Could you check a few things on this model? Use its own coordinates, in mm. Face numbers are marked on the shaded views. A direction names the side the tool comes from. Give positions to 0.01 mm unless a question says otherwise; leave off trailing zeros. Loops run counter-clockwise (first coordinate to the right, second up) from the corner with the lowest first, then second, coordinate; pieces in that order, holes last. Notation, with made-up numbers: (-7.5, -22.5) - (33.5, -22.5) arc R10 cw to (33.5, -13.5) - close; hole circle Ø11 at (38.5, 61.5). An arc over 180 degrees is marked (long way). Answer in a Markdown table with one row per item. Add a question column.
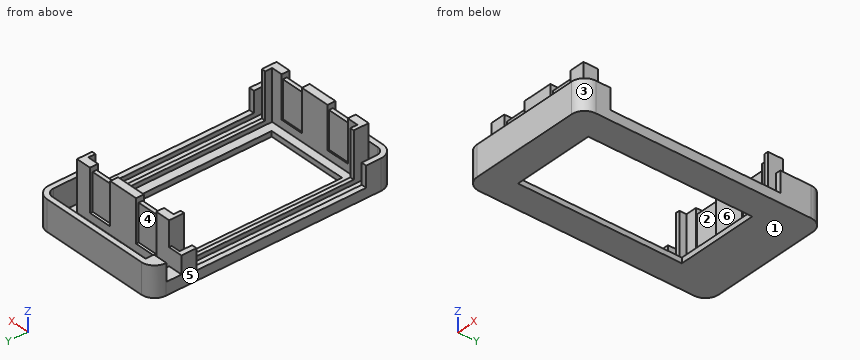
```python
from build123d import *

# Parameters (mm, degrees)
PAD_DEPTH       = 11.5
POCKET_DEPTH    = 9.5
PAD001_DEPTH    = 19
SKETCH003_W     = 5.8
SKETCH003_H     = 6.7
POCKET001_DEPTH = 6
SKETCH004_W     = 9
SKETCH004_H     = 76
POCKET002_DEPTH = 2
SKETCH005_W     = 9
SKETCH005_H     = 71
SKETCH005_H_2   = 1
POCKET003_DEPTH = 14
SKETCH006_W     = 31.339315
SKETCH006_H     = 62.470386
POCKET004_DEPTH = 5
SKETCH007_W     = 64.656841
SKETCH007_H     = 18.636995
POCKET005_DEPTH = 75


with BuildPart() as part:
    # Sketch → Pad (new body)
    with BuildSketch(Plane.XY):
        with BuildLine():
            Line((0, 5), (0, 87))
            ThreePointArc((5, 92), (1.464466, 90.535534), (0, 87))
            Line((5, 92), (47, 92))
            ThreePointArc((52, 87), (50.535534, 90.535534), (47, 92))
            Line((52, 87), (52, 5))
            ThreePointArc((47, 0), (50.535534, 1.464466), (52, 5))
            Line((47, 0), (5, 0))
            ThreePointArc((0, 5), (1.464466, 1.464466), (5, 0))
        make_face()
    extrude(amount=PAD_DEPTH)

    # Sketch001 → Pocket (cut)
    with BuildSketch(Plane.XY.offset(11.5)):
        with BuildLine():
            Line((2, 5), (2, 80))
            Line((2, 80), (5.5, 80))
            Line((5.5, 80), (5.5, 90))
            Line((5.5, 90), (47, 90))
            ThreePointArc((50, 87), (49.12132, 89.12132), (47, 90))
            Line((50, 87), (50, 5))
            ThreePointArc((47, 2), (49.12132, 2.87868), (50, 5))
            Line((47, 2), (5, 2))
            ThreePointArc((2, 5), (2.87868, 2.87868), (5, 2))
        make_face()
    extrude(amount=-POCKET_DEPTH, mode=Mode.SUBTRACT)

    # Sketch002 → Pad001 (new body)
    with BuildSketch(Plane.XY.offset(2)):
        Polygon((5.5, 5), (26, 5), (46.5, 5), (46.5, 81), (5.5, 81), align=None)
        Polygon((7, 78), (45, 78), (45, 8), (26, 8), (7, 8), align=None, mode=Mode.SUBTRACT)
    extrude(amount=PAD001_DEPTH)

    # Sketch003 → Pocket001 (cut)
    with BuildSketch(Plane(origin=(0, 0, 0), x_dir=(0, -1, 0), z_dir=(-1, 0, 0))):
        with Locations((-83.9, 8.15)):
            Rectangle(SKETCH003_W, SKETCH003_H)
    extrude(amount=-POCKET001_DEPTH, mode=Mode.SUBTRACT)

    # Sketch004 → Pocket002 (cut)
    with BuildSketch(Plane.XY.offset(21)):
        with Locations((15.75, 43)):
            Rectangle(SKETCH004_W, SKETCH004_H)
        with Locations((36.25, 43)):
            Rectangle(SKETCH004_W, SKETCH004_H)
    extrude(amount=-POCKET002_DEPTH, mode=Mode.SUBTRACT)

    # Sketch005 → Pocket003 (cut)
    with BuildSketch(Plane.XY.offset(19)):
        with Locations((15.75, 43)):
            Rectangle(SKETCH005_W, SKETCH005_H)
        with Locations((36.25, 43)):
            Rectangle(SKETCH005_W, SKETCH005_H)
        with Locations((15.75, 80.5)):
            Rectangle(SKETCH005_W, SKETCH005_H_2)
        with Locations((36.25, 80.5)):
            Rectangle(SKETCH005_W, SKETCH005_H_2)
        with Locations((15.75, 5.5)):
            Rectangle(SKETCH005_W, SKETCH005_H_2)
        with Locations((36.25, 5.5)):
            Rectangle(SKETCH005_W, SKETCH005_H_2)
    extrude(amount=-POCKET003_DEPTH, mode=Mode.SUBTRACT)

    # Sketch006 → Pocket004 (cut)
    with BuildSketch(Plane.XY.offset(2)):
        with Locations((25.891194, 42.313818)):
            Rectangle(SKETCH006_W, SKETCH006_H)
    extrude(amount=-POCKET004_DEPTH, mode=Mode.SUBTRACT)

    # Sketch007 → Pocket005 (cut)
    with BuildSketch(Plane(origin=(0, 0, 0), x_dir=(0, -1, 0), z_dir=(-1, 0, 0))):
        with Locations((-42.974649, 12.963171)):
            Rectangle(SKETCH007_W, SKETCH007_H)
    extrude(amount=-POCKET005_DEPTH, mode=Mode.SUBTRACT)


solid = part.part
```
(1) I want a section at D-D on y = 85.5. Please give me the cut outline in (x, z).
(2) I want a section at A-A on y = 69. Please give me the cut outline in (x, z), then the cut area to 3 significant figures.
(3) I want a section at B-B on x = 38.5. Please give me the cut outline in (y, z).
(4) We'd pull the mould along Y, two halves only. Please class the marked faces 3, 4, 5 and 6: pulls with the +Y half, pulls with the -Y half, needs draft (parallel to the pull), parting line crosses it, or undercut.
(5) Please list where these lines run through material, in increasing order: line 1 (Y direction, x = 9, z = 2.75); line 2 (X direction, y = 10, z = 5); line 3 (Y direction, x = 18.5, z = 10.75).
(6) I want a section at C-C on x = 44. Please give me the cut outline in (y, z).
(7) For pin 1 Ø1.2 at (x, y) = (35.5, 79.5) entering from +Z; pin 2 Ø0.6 at (x, y) = (51, 54) entering from +Z; pin 3 Ø4 at (x, z) = (21.5, 15) entering from -Y; pin 4 Ø5 at (x, y) = (20, 81) entering from +Z, each with a flat end and sliding along its axis, tell me the tip position at first contact or that it passes through.
(8) On a 3-axis mill with a long thin cutter (end or side, diameter ignored), from which of +Z, -Z, +X, -X, +Y, -Y can I reach the whole of each face in a straight line? I mean the marked faces 1 and 2. Say none if no direction works.
Reported:
| question | item | result |
|---|---|---|
| 1 | outline | (0, 0) - (52, 0) - (52, 11.5) - (50, 11.5) - (50, 2) - (5.5, 2) - (5.5, 4.8) - (0, 4.8) - close |
| 2 | outline | (0, 0) - (10.22, 0) - (10.22, 2) - (7, 2) - (7, 3.64) - (5.5, 3.64) - (5.5, 2) - (2, 2) - (2, 3.64) - (0, 3.64) - close; (41.56, 0) - (52, 0) - (52, 3.64) - (50, 3.64) - (50, 2) - (46.5, 2) - (46.5, 3.64) - (45, 3.64) - (45, 2) - (41.56, 2) - close |
| 2 | area | 52.8 mm² |
| 3 | outline | (0, 0) - (11.08, 0) - (11.08, 2) - (8, 2) - (8, 5) - (7.5, 5) - (7.5, 19) - (6, 19) - (6, 5) - (5, 5) - (5, 2) - (2, 2) - (2, 11.5) - (0, 11.5) - close; (73.55, 0) - (92, 0) - (92, 11.5) - (90, 11.5) - (90, 2) - (81, 2) - (81, 5) - (80, 5) - (80, 19) - (78.5, 19) - (78.5, 5) - (78, 5) - (78, 2) - (73.55, 2) - close |
| 4 | face 3 | pulls with the -Y half |
| 4 | face 4 | undercut |
| 4 | face 5 | needs draft |
| 4 | face 6 | undercut |
| 5 | line 1 | 0 to 2, 5 to 8, 78 to 81, 90 to 92 |
| 5 | line 2 | 0 to 2, 5.5 to 7, 45 to 46.5, 50 to 52 |
| 5 | line 3 | 0 to 2, 6 to 7.5, 78.5 to 80, 90 to 92 |
| 6 | outline | (0, 0) - (92, 0) - (92, 11.5) - (90, 11.5) - (90, 2) - (81, 2) - (81, 21) - (78, 21) - (78, 2) - (8, 2) - (8, 21) - (5, 21) - (5, 2) - (2, 2) - (2, 11.5) - (0, 11.5) - close |
| 7 | pin 1 | z = 19 |
| 7 | pin 2 | z = 3.64 |
| 7 | pin 3 | y = 5 |
| 7 | pin 4 | z = 21 |
| 8 | face 1 | -Z, +X, -X, +Y, -Y |
| 8 | face 2 | +Z |
